Autodesk Inventor part; units mm, degrees
ref_plane "YZ Plane" through (0, 0, 0) normal (1, 0, 0) x (0, 1, 0)
ref_plane "XZ Plane" through (0, 0, 0) normal (0, 1, 0) x (-1, 0, 0)
ref_plane "XY Plane" through (0, 0, 0) normal (0, 0, 1) x (1, 0, 0)
sketch "Sketch1" plane through (0, 0, 0) normal (0, 0, 1) x (1, 0, 0)
  line L0 (-58, -50) -> (-58, 50) construction
  line L1 (-58, -50) -> (58, -50) construction
  line L2 (58, 50) -> (58, -50) construction
  line L3 (58, 50) -> (-58, 50) construction
  line L4 (-48.8, -35) -> (-48.8, -43.5) construction
  arc A0 (-55.2, -43.5) -> (-48.8, -43.5) centre (-52, -43.5) ccw construction
  line L5 (-55.2, -43.5) -> (-55.2, -35) construction
  arc A1 (-48.8, -35) -> (-55.2, -35) centre (-52, -35) ccw construction
  line L6 (55.2, -35) -> (55.2, -43.5) construction
  arc A2 (48.8, -43.5) -> (55.2, -43.5) centre (52, -43.5) ccw construction
  line L7 (48.8, -43.5) -> (48.8, -35) construction
  arc A3 (55.2, -35) -> (48.8, -35) centre (52, -35) ccw construction
  circle A4 centre (10.25, -35) radius 3.2 construction
  circle A5 centre (-10.25, -35) radius 3.2 construction
  circle A6 centre (-10.25, 35) radius 3.2 construction
  circle A7 centre (10.25, 35) radius 3.2 construction
  line L8 (-55.2, 35) -> (-55.2, 43.5) construction
  arc A8 (-48.8, 43.5) -> (-55.2, 43.5) centre (-52, 43.5) ccw construction
  line L9 (-48.8, 43.5) -> (-48.8, 35) construction
  arc A9 (-55.2, 35) -> (-48.8, 35) centre (-52, 35) ccw construction
  circle A10 centre (-52, 7.125) radius 3.2 construction
  line L10 (-7.05, -7.125) -> (-7.05, -15.625) construction
  arc A11 (-13.45, -15.625) -> (-7.05, -15.625) centre (-10.25, -15.625) ccw construction
  line L11 (-13.45, -15.625) -> (-13.45, -7.125) construction
  arc A12 (-7.05, -7.125) -> (-13.45, -7.125) centre (-10.25, -7.125) ccw construction
  circle A13 centre (52, -7.125) radius 3.2 construction
  circle A14 centre (-52, -7.125) radius 3.2 construction
  line L12 (13.45, -7.125) -> (13.45, -15.625) construction
  arc A15 (7.05, -15.625) -> (13.45, -15.625) centre (10.25, -15.625) ccw construction
  line L13 (7.05, -15.625) -> (7.05, -7.125) construction
  arc A16 (13.45, -7.125) -> (7.05, -7.125) centre (10.25, -7.125) ccw construction
  circle A17 centre (52, 7.125) radius 3.2 construction
  line L14 (13.45, 15.625) -> (13.45, 7.125) construction
  arc A18 (7.05, 7.125) -> (13.45, 7.125) centre (10.25, 7.125) ccw construction
  line L15 (7.05, 7.125) -> (7.05, 15.625) construction
  arc A19 (13.45, 15.625) -> (7.05, 15.625) centre (10.25, 15.625) ccw construction
  line L16 (55.2, 43.5) -> (55.2, 35) construction
  arc A20 (48.8, 35) -> (55.2, 35) centre (52, 35) ccw construction
  line L17 (48.8, 35) -> (48.8, 43.5) construction
  arc A21 (55.2, 43.5) -> (48.8, 43.5) centre (52, 43.5) ccw construction
  line L18 (-7.05, 15.625) -> (-7.05, 7.125) construction
  arc A22 (-13.45, 7.125) -> (-7.05, 7.125) centre (-10.25, 7.125) ccw construction
  line L19 (-13.45, 7.125) -> (-13.45, 15.625) construction
  arc A23 (-7.05, 15.625) -> (-13.45, 15.625) centre (-10.25, 15.625) ccw construction
  line L20 (60, 50) -> (58, 50) construction
  line L21 (58, 50) -> (58, -50) construction
  line L22 (58, -50) -> (60, -50) construction
  line L23 (60, -50) -> (60, 50) construction
  line L24 (-60, -50) -> (-58, -50) construction
  line L25 (-58, -50) -> (-58, 50) construction
  line L26 (-58, 50) -> (-60, 50) construction
  line L27 (-60, 50) -> (-60, -50) construction
  circle A24 centre (-52, 43.5) radius 3.2
  circle A25 centre (-10.25, 15.625) radius 3.2
  circle A26 centre (52, 43.5) radius 3.2
  circle A27 centre (-52, -43.5) radius 3.2
  circle A28 centre (-52, 7.125) radius 3.2
  circle A29 centre (-52, -7.125) radius 3.2
  circle A30 centre (-10.25, -15.625) radius 3.2
  circle A31 centre (-10.25, -35) radius 3.2
  circle A32 centre (-10.25, 35) radius 3.2
  line L28 (-60, 50) -> (-60, -50)
  line L29 (-60, -50) -> (-35, -50)
  line L30 (0, -15) -> (0, 15)
  line L31 (-60, 50) -> (-35, 50)
  circle A33 centre (-10.25, 7.125) radius 3.2
  circle A34 centre (-10.25, -7.125) radius 3.2
  line L32 (-35, 50) -> (-25.2404, 40.2404)
  line L33 (-25.2404, 40.2404) -> (-25.2404, 15)
  line L34 (-35, -50) -> (-25.2404, -40.2404)
  line L35 (-25.2404, -40.2404) -> (-25.2404, -15)
  line L36 (-25.2404, -15) -> (0, -15)
  line L37 (-25.2404, 15) -> (0, 15)
  point P0 (0, 0)
  point P1 (0, 0)
  dimension "d13" = 35
  dimension "d19" = 135
  dimension "d20" = 135
  dimension "d21" = 30
extrude "Extrusion1" add sketch "Sketch1" along normal blind 18 contours L37 A25 | A25 L37 L30 L36 A30 L35 L34 L29 L28 L31 L32 L33 | L36 A30 picked at (-10.8738, 14.3431) picked at (-10.6405, -14.2157)
sketch "Sketch4" plane through (-60, -50, 0) normal (-1, 0, 0) x (0, 0, 1)
  line L0 (16, 100) -> (16, 0)
  line L1 (16, 100) -> (0, 100)
  line L2 (0, 88) -> (0, 100)
  arc A0 (0, 72) -> (0, 88) centre (0, 80) ccw
  line L3 (0, 62.5) -> (0, 72)
  arc A1 (0, 37.5) -> (0, 62.5) centre (0, 50) ccw
  line L4 (0, 28) -> (0, 37.5)
  arc A2 (0, 12) -> (0, 28) centre (0, 20) ccw
  line L5 (0, 0) -> (0, 12)
  line L6 (16, 0) -> (0, 0)
  line L7 (-16, 0) -> (-16, 100)
  line L8 (-16, 0) -> (0, 0)
  line L9 (0, 12) -> (0, 0)
  arc A3 (0, 28) -> (0, 12) centre (0, 20) ccw
  line L10 (0, 37.5) -> (0, 28)
  arc A4 (0, 62.5) -> (0, 37.5) centre (0, 50) ccw
  line L11 (0, 72) -> (0, 62.5)
  arc A5 (0, 88) -> (0, 72) centre (0, 80) ccw
  line L12 (0, 100) -> (0, 88)
  line L13 (-16, 100) -> (0, 100)
  circle A6 centre (0, 50) radius 3.3
  point P0 (0, 50)
extrude "Extrusion4" cut sketch "Sketch4" against normal through all contours A0 A5 | A3 A2 | A6
chamfer "Chamfer3" distance 2 angle 45 4 edges at (-60, 0, 18) (0, 0, 18) (-25.2404, -27.6202, 18) (-25.2404, 27.6202, 18)
chamfer "Chamfer4" distance 5 angle 45 4 edges at (-25.2404, 15, 8) (-25.2404, -15, 8) (0, -15, 8) (0, 15, 8)
properties part number "AX_XY" material "PC/ABS Plastic"
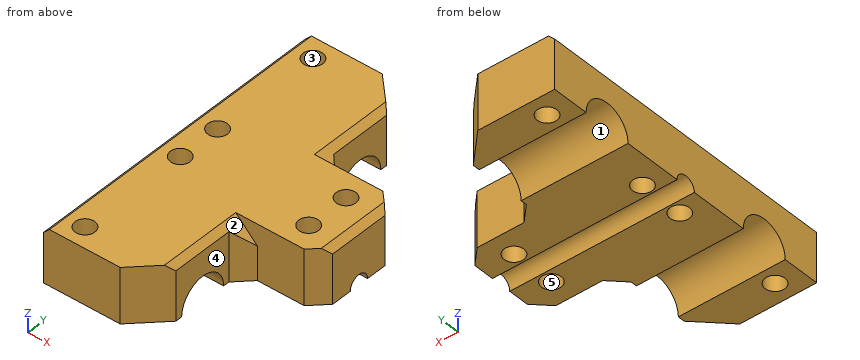
The model under review builds one solid part; all positions refer to its coordinate system, in mm. Face numbers are marked on the shaded views. A direction names the side the tool comes from. Round coordinates to 2 decimals unless told otherwise and drop trailing zeros. Loops run counter-clockwise (first coordinate to the right, second up) from the corner with the lowest first, then second, coordinate; pieces in that order, holes last. Notation, with made-up numbers: M 62,17 L 116,17 A17 cw 116,29 Z; hole C 1,21 d7. An arc over 180 degrees is marked long. Answer as CSV lines item,"result".
1. To check wall thickness, follow L1, parallel to X at y = 7.5, z = 12.5; L2, parallel to Y at x = -34, z = 6.5; L3, parallel to Y at x = -10.25, z = 8 (3 decimals). State the ranges of each line that lie inside material, in increasing order. Write a range as [from, to].
Outcome:
L1,"x = [-60, -55.18], [-48.82, -13.43], [-7.07, 0]"
L2,"y = [-49, -34.66], [-25.34, 25.34], [34.66, 49]"
L3,"y = [-15, -10.325], [-3.925, 3.925], [10.325, 15]"
2. We need section A-A (y = 43.5). Give the boundary of the cut face in (x, z).
Outcome:
outline,"M -60,0 L -55.2,0 L -55.2,18 L -58,18 L -60,16 Z; M -48.8,0 L -28.5,0 L -28.5,18 L -48.8,18 Z"
3. We need section C-C (x = -52). Give the boundary of the cut face in (y, z) (3 decimals), plus the area to 3 significant figures.
Outcome:
outline,"M -50,0 L -46.7,0 L -46.7,18 L -50,18 Z; M -40.3,0 L -38,0 A8 cw -22,0 L -10.325,0 L -10.325,18 L -40.3,18 Z; M -3.925,0 L -3.3,0 A3.3 cw 3.3,0 L 3.925,0 L 3.925,18 L -3.925,18 Z; M 10.325,0 L 22,0 A8 cw 38,0 L 40.3,0 L 40.3,18 L 10.325,18 Z; M 46.7,0 L 50,0 L 50,18 L 46.7,18 Z"
area,"1,120 mm2"
4. We need section D-D (y = -9). Give the boundary of the cut face in (x, z), plus the area to 3 significant figures.
Outcome:
outline,"M -60,0 L -54.59,0 L -54.59,18 L -58,18 L -60,16 Z; M -49.41,0 L -12.84,0 L -12.84,18 L -49.41,18 Z; M -7.66,0 L 0,0 L 0,16 L -2,18 L -7.66,18 Z"
area,"889 mm2"
5. Insertion check: pin 1 Ø9 at (x, z) = (-20.5, 4.5) entering from +Y; pin 2 Ø1 at (y, z) = (-21.5, 12.5) entering from +X; pin 3 Ø6 at (x, z) = (-21, 10) entering from +Y. Each pin has a flat end and moves straight along its axis. Give the tip position at first contact, or say it passes through.
Outcome:
pin 1,"stops at y = 19.76"
pin 2,"stops at x = -25.24"
pin 3,"stops at y = 18.76"
6. We need section B-B (x = -10.25). Give the boundary of the cut face in (y, z) (3 decimals), plus the area to 3 significant figures.
Outcome:
outline,"M -15,0 L -10.325,0 L -10.325,18 L -15,18 Z; M -3.925,0 L -3.3,0 A3.3 cw 3.3,0 L 3.925,0 L 3.925,18 L -3.925,18 Z; M 10.325,0 L 15,0 L 15,18 L 10.325,18 Z"
area,"292 mm2"
7. Draft analysis for pull direction X (two halves, no side actions). For the marked faces 1, 2 and 3, state which applies: pulls with the +X half, pulls with the -X half, needs draft (parallel to the pull), parting line crosses it, or undercut.
Outcome:
face 1,"needs draft"
face 2,"pulls with the +X half"
face 3,"undercut"
8. For the marked faces 4 and 5, list the 3-axis set-ups (+Z, -Z, +X, -X, +Y, -Y) from which the entire face can be reached by the end or side of a thin tool; tool diameter is ignored.
Outcome:
face 4,"+Z, -Z, +X, -Y"
face 5,"+Z, -Z"
